Geometry check sheet. Reference: the model listing, model coordinates, mm. Face numbers are marked on the shaded views. Coordinates: 2 decimals unless noted, no trailing zeros. Write each loop counter-clockwise with the first axis right and the second up, starting at its lowest first coordinate (ties: lowest second). Pieces come first, ordered by that corner, then holes.
from build123d import *

# Parameters (mm, degrees)
IZIM1_R                     = 15
Y_KSEKLIK_EKSTR_ZYON1_DEPTH = 44
IZIM3_R                     = 10
KES_EKSTR_ZYON1_DEPTH       = 30
IZIM4_R                     = 2
KES_EKSTR_ZYON2_DEPTH       = 60


with BuildPart() as part:
    # Çizim1 → Yükseklik-Ekstrüzyon1 (new body)
    with BuildSketch(Plane.XY):
        Circle(IZIM1_R)
    extrude(amount=Y_KSEKLIK_EKSTR_ZYON1_DEPTH)

    # Çizim3 → Kes-Ekstrüzyon1 (cut)
    with BuildSketch(Plane.XY.offset(44)):
        Circle(IZIM3_R)
    extrude(amount=-KES_EKSTR_ZYON1_DEPTH, mode=Mode.SUBTRACT)

    # Çizim4 → Kes-Ekstrüzyon2 (cut)
    with BuildSketch(Plane(origin=(0, 15, 0), x_dir=(1, 0, 0), z_dir=(0, 1, 0))):
        with Locations(Location((0, -36, 0), (0, 0, 270))):
            Circle(IZIM4_R)
    extrude(amount=-KES_EKSTR_ZYON2_DEPTH, mode=Mode.SUBTRACT)


solid = part.part
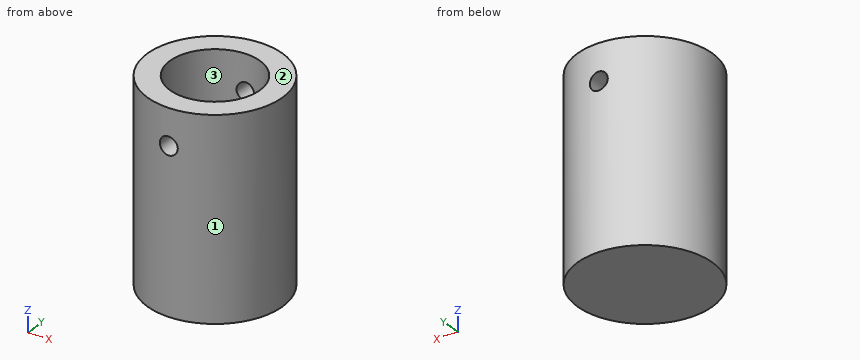
1. Sectioned sample at B-B, the plane z = 36. Record the boundary of the cut face in (x, y).
Computed values:
outline: (-2, -14.87) - (-2, -9.8) arc R10 cw to (-2, 9.8) - (-2, 14.87) arc R15 ccw to start; (2, -14.87) arc R15 ccw to (2, 14.87) - (2, 9.8) arc R10 cw to (2, -9.8) - close
2. Sectioned sample at D-D, the plane y = -12. Record the boundary of the cut face in (x, z).
Computed values:
outline: (-9, 0) - (9, 0) - (9, 44) - (-9, 44) - close; hole circle Ø4 at (0, 36)
3. Gauge pin test, flat ends, axial feed: pin 1 Ø5 at (x, z) = (12, 26.5) entering from +Y; pin 2 Ø10 at (x, y) = (-4.5, -1.5) entering from +Z; pin 3 Ø5 at (x, z) = (-6.5, 36.5) entering from +Y; pin 4 Ø3 at (x, z) = (0, 36) entering from +Y. Record the tip position at first contact, or that the pin passes through.
Computed values:
pin 1: stops at y = 11.61
pin 2: stops at z = 14
pin 3: stops at y = 14.46
pin 4: passes through
4. Sectioned sample at A-A, the plane x = 0. Record the boundary of the cut face in (y, z), and give its area (3 significant figures).
Computed values:
outline: (-15, 0) - (15, 0) - (15, 34) - (10, 34) - (10, 14) - (-10, 14) - (-10, 34) - (-15, 34) - close; (-15, 38) - (-10, 38) - (-10, 44) - (-15, 44) - close; (10, 38) - (15, 38) - (15, 44) - (10, 44) - close
area: 680 mm2
5. Sectioned sample at C-C, the plane y = 0. Record the boundary of the cut face in (x, z), and give its area (3 significant figures).
Computed values:
outline: (-15, 0) - (15, 0) - (15, 44) - (10, 44) - (10, 14) - (-10, 14) - (-10, 44) - (-15, 44) - close
area: 720 mm2
6. Thickness scan on line 1 along Z through (x, y) = (0, -11); line 2 along Z through (x, y) = (5, 0); line 3 along X through (y, z) = (-7, 34). Record the ranges inside material, lowest first.
Computed values:
line 1: z = 0 to 34, 38 to 44
line 2: z = 0 to 14
line 3: x = -13.27 to -7.14, 7.14 to 13.27
7. Draft check along X on the marked faces 1, 2 and 3. Enter one of: released by +X, released by -X, zero draft, split by the parting line, or undercut.
Computed values:
face 1: split by the parting line
face 2: zero draft
face 3: undercut
